Source: CAD feature listing. Evaluate the final solid. Frame: model axes, mm. A direction names the side the tool comes from. Give positions to 0.01 mm unless a question says otherwise; leave off trailing zeros. Order: outer loops, then holes, each group sorted by start corner. A loop starts at its lowest first (then second) coordinate and runs counter-clockwise, first axis right, second up. Notation, with made-up numbers: (75, -16) -> (96, -16) arc R30 cw to (96, 15) -> close; hole circle Ø3 at (47, -24). An arc over 180 degrees is marked (long way). Answer in a Markdown table with one row per item.
```python
from build123d import *

# Parameters (mm, degrees)
CROQUIS1_R              = 14
CROQUIS1_W              = 14.155779923
CROQUIS1_H              = 14.6
SALIENTE_EXTRUIR1_DEPTH = 19
CROQUIS2_R              = 4.5
SALIENTE_EXTRUIR2_DEPTH = 1.5
CROQUIS3_R              = 2.5
SALIENTE_EXTRUIR3_DEPTH = 2.5
SALIENTE_EXTRUIR4_DEPTH = 6
CROQUIS5_W              = 18.5
CROQUIS5_H              = 1.5
CORTAR_EXTRUIR3_DEPTH   = 50
CROQUIS6_R              = 2.5
SALIENTE_EXTRUIR5_DEPTH = 5


with BuildPart() as part:
    # Croquis1 → Saliente-Extruir1 (new body)
    with BuildSketch(Plane(origin=(0, 0, 0), x_dir=(1, 0, 0), z_dir=(0, 1, 0))):
        Circle(CROQUIS1_R)
        with Locations((9.922110038, 0)):
            Rectangle(CROQUIS1_W, CROQUIS1_H)
    extrude(amount=SALIENTE_EXTRUIR1_DEPTH)

    # Croquis2 → Saliente-Extruir2 (add)
    with BuildSketch(Plane(origin=(0, 19, 0), x_dir=(1, 0, 0), z_dir=(0, 1, 0))):
        with Locations((-8, 0)):
            Circle(CROQUIS2_R)
    extrude(amount=SALIENTE_EXTRUIR2_DEPTH)

    # Croquis3 → Saliente-Extruir3 (add)
    with BuildSketch(Plane(origin=(0, 20.5, 0), x_dir=(1, 0, 0), z_dir=(0, 1, 0))):
        with Locations((-8, 0)):
            Circle(CROQUIS3_R)
    extrude(amount=SALIENTE_EXTRUIR3_DEPTH)

    # Croquis4 → Saliente-Extruir4 (add)
    with BuildSketch(Plane(origin=(0, 23, 0), x_dir=(1, 0, 0), z_dir=(0, 1, 0))):
        with BuildLine():
            Line((-9.5, 2), (-9.5, -2))
            ThreePointArc((-9.5, -2), (-8, -2.5), (-6.5, -2))
            Line((-6.5, -2), (-6.5, 2))
            ThreePointArc((-6.5, 2), (-8, 2.5), (-9.5, 2))
        make_face()
    extrude(amount=SALIENTE_EXTRUIR4_DEPTH)

    # Croquis5 → Cortar-Extruir3 (cut)
    with BuildSketch(Plane(origin=(17, 0, 0), x_dir=(0, 0, -1), z_dir=(1, 0, 0))):
        with Locations((-4.75, 19.75)):
            Rectangle(CROQUIS5_W, CROQUIS5_H)
        Polygon((4.5, 19), (-14, 19), (-14, 0), (14, 0), (14, 19), align=None)
    extrude(amount=-CORTAR_EXTRUIR3_DEPTH, mode=Mode.SUBTRACT)

    # Croquis6 → Saliente-Extruir5 (add)
    with BuildSketch(Plane.XZ.offset(-20.5)):
        with Locations((-8, 0)):
            Circle(CROQUIS6_R)
    extrude(amount=SALIENTE_EXTRUIR5_DEPTH)


solid = part.part
```
(1) Access query for faces 1 (the flat face through (-6, 23, 0)), 2 (the flat face through (-8, 29, 0)), 3 (the flat face through (-10, 23, 0)). Directions: +Z, -Z, +X, -X, +Y, -Y. A direction counts if a zero-diameter tool reaches every point of the face in a straight line with its end or side. Return the directions, or none.
A:
| item | result |
|---|---|
| face 1 | +Z, -Z, +X, +Y |
| face 2 | +Z, -Z, +X, -X, +Y |
| face 3 | +Z, -Z, -X, +Y |
(2) Section query D-D (z = 1.8). Return the cut outline in (x, y).
A:
| item | result |
|---|---|
| outline | (-9.73, 15.5) -> (-6.27, 15.5) -> (-6.27, 23) -> (-6.5, 23) -> (-6.5, 29) -> (-9.5, 29) -> (-9.5, 23) -> (-9.73, 23) -> close |
(3) Section query B-B (y = 23.25). Return the cut outline in (x, z).
A:
| item | result |
|---|---|
| outline | (-9.5, -2) arc R2.5 ccw to (-6.5, -2) -> (-6.5, 2) arc R2.5 ccw to (-9.5, 2) -> close |
(4) Section query A-A (z = 0). Return the cut outline in (x, y).
A:
| item | result |
|---|---|
| outline | (-10.5, 15.5) -> (-5.5, 15.5) -> (-5.5, 23) -> (-6.5, 23) -> (-6.5, 29) -> (-9.5, 29) -> (-9.5, 23) -> (-10.5, 23) -> close |
(5) Section query C-C (x = -9.15). Return the cut outline in (y, z).
A:
| item | result |
|---|---|
| outline | (15.5, -2.22) -> (29, -2.22) -> (29, 2.22) -> (15.5, 2.22) -> close |
(6) First-contact query: pin 1 Ø3 at (x, y) = (-6.5, 23.5) entering from -Z; pin 2 Ø3 at (y, z) = (25, 0) entering from +X; pin 3 Ø1 at (y, z) = (23, -1) entering from +X; pin 4 Ø3 at (y, z) = (25, 0) entering from -X. Flat tips, straight axial feed; report the tip coordinate or a pass-through.
A:
| item | result |
|---|---|
| pin 1 | stops at z = -2.5 |
| pin 2 | stops at x = -6.5 |
| pin 3 | stops at x = -5.55 |
| pin 4 | stops at x = -9.5 |
(7) Ray query, probe 1 along X at (y, z) = (25.75, 1.6); probe 2 along Y at (x, z) = (-9.6, 0.2); probe 3 along Z at (x, y) = (-9, 27). Return the intervals inside material, ascending.
A:
| item | result |
|---|---|
| probe 1 | x = -9.5 to -6.5 |
| probe 2 | y = 15.5 to 23 |
| probe 3 | z = -2.29 to 2.29 |
